Verification items for the finished model (mm, model axes). Coordinates: 2 decimals unless noted, no trailing zeros. Write each loop counter-clockwise with the first axis right and the second up, starting at its lowest first coordinate (ties: lowest second). Pieces come first, ordered by that corner, then holes. Notation, with made-up numbers: (-20, 56) -> (36, 56) arc R22 cw to (36, 81) -> close; hole circle Ø11 at (4, -24). An arc over 180 degrees is marked (long way). Answer in a Markdown table with one row per item.
```python
from build123d import *

# Parameters (mm, degrees)
SKETCH1_W             = 101.6
SKETCH1_H             = 158.75
BOSS_EXTRUDE1_DEPTH   = 6.35
F_6_CLEARANCE_HOLE1_D = 3.7973


with BuildPart() as part:
    # Sketch1 → Boss-Extrude1 (new body)
    with BuildSketch(Plane(origin=(0, 0, 0), x_dir=(0, 0, -1), z_dir=(1, 0, 0))):
        Rectangle(SKETCH1_W, SKETCH1_H)
    extrude(amount=BOSS_EXTRUDE1_DEPTH)

    # #6 Clearance Hole1 (through all)
    with Locations(Plane.ZY):
        with Locations((-47.625, 53.975), (-20.6375, 76.2), (26.9875, 76.2), (26.9875, -76.2), (-20.6375, -76.2), (-47.625, -53.975)):
            Hole(F_6_CLEARANCE_HOLE1_D / 2)


solid = part.part
```
1. Go/stop test with a flat-tipped pin: pin 1 (2.5 mm diameter, centred on y = -76.2, z = -20.64, fed in from +X). Record where the tip stops, or that it passes through.
Findings below:
| item | result |
|---|---|
| pin 1 | passes through |
2. Sectioned sample at A-A, the plane y = 76.2. Record the cut outline in (x, z), and give its area (3 significant figures).
Findings below:
| item | result |
|---|---|
| outline | (0, -50.8) -> (6.35, -50.8) -> (6.35, -22.54) -> (0, -22.54) -> close; (0, -18.74) -> (6.35, -18.74) -> (6.35, 25.09) -> (0, 25.09) -> close; (0, 28.89) -> (6.35, 28.89) -> (6.35, 50.8) -> (0, 50.8) -> close |
| area | 597 mm² |
3. Material ranges on probe 1 along Z at (x, y) = (4, 76.2); probe 2 along Y at (x, z) = (5.5, 28.5) (3 decimals); probe 3 along Z at (x, y) = (1.75, -54.5), recorded low to high. Write a range as from..to.
Findings below:
| item | result |
|---|---|
| probe 1 | z = -50.8..-22.54, -18.74..25.09, 28.89..50.8 |
| probe 2 | y = -79.375..-77.348, -75.052..75.052, 77.348..79.375 |
| probe 3 | z = -50.8..-49.45, -45.8..50.8 |
4. Release check for a two-part mould opening along Y. For faces 1 (the face through (3, 79.375, 1)), 2 (the face through (0, 1, 1)), 3 (the face through (3.22, -55.13, -46.12)) record: released by +Y, released by -Y, zero draft, split by the parting line, or undercut.
Findings below:
| item | result |
|---|---|
| face 1 | released by +Y |
| face 2 | zero draft |
| face 3 | undercut |
